Geometry check sheet. Reference: the model listing, model coordinates, mm. A direction names the side the tool comes from. Coordinates: 2 decimals unless noted, no trailing zeros. Write each loop counter-clockwise with the first axis right and the second up, starting at its lowest first coordinate (ties: lowest second). Pieces come first, ordered by that corner, then holes. Notation, with made-up numbers: (-20.75, 72.25) -> (38.25, 72.25) arc R24 cw to (38.25, 105.25) -> close; hole circle Ø4 at (10, -15). An arc over 180 degrees is marked (long way). Answer in a Markdown table with one row per item. Add a question column.
Q1. Thickness scan on line 1 (Z direction, x = 13, y = -44); line 2 (Z direction, x = -9, y = -17); line 3 (X direction, y = -8.5, z = 63). Record the ranges inside material, lowest first.
Q2. Tool access check on faces 1 (the face through (9.934, -49, 29)), 2 (the face through (29.926, -25, 20)), 3 (the face through (-20.112, -49, 12)). Record the directions out of +Z, -Z, +X, -X, +Y, -Y that give a thin tool (end or side, any length) a straight path to the whole face; none if there is none.
Q3. Section check D-D, the plane x = -7. Record the boundary of the cut face in (y, z), and give its area (3 significant figures).
Q4. Section check C-C, the plane z = 60.5. Record the boundary of the cut face in (x, y).
Q5. Release check for a two-part mould opening along Z. For faces 4 (the face through (15.172, -24.65, 54.702)), 5 (the face through (0, -50, 28)), 6 (the face through (13.811, -49, 37)) record: pulls with the +Z half, pulls with the -Z half, needs draft (parallel to the pull), parting line crosses it, or undercut.
Q6. Gauge pin test, flat ends, axial feed: P1, Ø2, axis at x = 17.5, z = 29, coming from the -Y side; P2, Ø1, axis at x = 9, y = -38, coming from the +Z side; P3, Ø1, axis at y = -43.5, z = 62.5, coming from the -X side. Record the tip position at first contact, or that the pin passes through.
Q7. Section check A-A, the plane y = -8. Record the boundary of the cut face in (x, z).
Q8. Section check B-B, the plane x = -18. Record the boundary of the cut face in (y, z), and give its area (3 significant figures).
```python
from build123d import *

# Parameters (mm, degrees)
PAD_DEPTH            = 50
SKETCH001_W          = 14.321759
SKETCH001_H          = 23.338661
POCKET_DEPTH         = 2
SKETCH004_W          = 3.777545
SKETCH004_H          = 5.566906
POCKET001_DEPTH      = 2
SKETCH005_W          = 3.988077
SKETCH005_H          = 5.534469
POCKET002_DEPTH      = 2
SKETCH006_W          = 3.743909
SKETCH006_H          = 5.941416
POCKET003_DEPTH      = 2
SKETCH007_W          = 4.200878
SKETCH007_H          = 5.837583
POCKET004_DEPTH      = 2
BODY_PLACEMENT_ANGLE = 90


with BuildPart() as part:
    # Sketch → Pad (new body)
    with BuildSketch(Plane.XY):
        Polygon((-30.008501, 0), (29.925684, 0), (29.925684, 39.928391), (0, 69.895485), (-30.008501, 40.105713), align=None)
    extrude(amount=PAD_DEPTH)

    # Sketch001 (on Face7 of Pad) → Pocket (cut)
    with BuildSketch(Plane.XY.offset(50)):
        with Locations((-12.951147, 11.66933)):
            Rectangle(SKETCH001_W, SKETCH001_H)
    extrude(amount=-POCKET_DEPTH, mode=Mode.SUBTRACT)

    # Sketch004 (on Face4 of Pocket) → Pocket001 (cut)
    with BuildSketch(Plane.XY.offset(50)):
        with Locations((11.92271, 37.153109)):
            Rectangle(SKETCH004_W, SKETCH004_H)
    extrude(amount=-POCKET001_DEPTH, mode=Mode.SUBTRACT)

    # Sketch005 (on Face4 of Pocket001) → Pocket002 (cut)
    with BuildSketch(Plane.XY.offset(50)):
        with Locations((18.594975, 37.152287)):
            Rectangle(SKETCH005_W, SKETCH005_H)
    extrude(amount=-POCKET002_DEPTH, mode=Mode.SUBTRACT)

    # Sketch006 (on Face4 of Pocket002) → Pocket003 (cut)
    with BuildSketch(Plane.XY.offset(50)):
        with Locations((11.805747, 28.857034)):
            Rectangle(SKETCH006_W, SKETCH006_H)
    extrude(amount=-POCKET003_DEPTH, mode=Mode.SUBTRACT)

    # Sketch007 (on Face4 of Pocket003) → Pocket004 (cut)
    with BuildSketch(Plane.XY.offset(50)):
        with Locations((18.480049, 28.816772)):
            Rectangle(SKETCH007_W, SKETCH007_H)
    extrude(amount=-POCKET004_DEPTH, mode=Mode.SUBTRACT)


with BuildPart() as part_1:
    # Body placement: moved
    add(part.part.rotate(Axis((0, 0, 0), (1, 0, 0)), BODY_PLACEMENT_ANGLE))


solid = part_1.part
```
Calculated:
| question | item | result |
|---|---|---|
| 1 | line 1 | z = 0 to 56.88 |
| 1 | line 2 | z = 0 to 60.96 |
| 1 | line 3 | x = -6.95 to 6.89 |
| 2 | face 1 | -Y |
| 2 | face 2 | +Z, -Z, +X, +Y, -Y |
| 2 | face 3 | -Z, -Y |
| 3 | outline | (-50, 23.34) -> (-48, 23.34) -> (-48, 0) -> (0, 0) -> (0, 62.95) -> (-50, 62.95) -> close |
| 3 | area | 3,100 mm² |
| 4 | outline | (-9.46, -50) -> (9.38, -50) -> (9.38, 0) -> (-9.46, 0) -> close |
| 5 | face 4 | pulls with the +Z half |
| 5 | face 5 | needs draft |
| 5 | face 6 | undercut |
| 6 | P1 | stops at y = -48 |
| 6 | P2 | stops at z = 61.38 |
| 6 | P3 | stops at x = -7.95 |
| 7 | outline | (-30.01, 0) -> (29.93, 0) -> (29.93, 39.93) -> (0, 69.9) -> (-30.01, 40.11) -> close |
| 8 | outline | (-50, 23.34) -> (-48, 23.34) -> (-48, 0) -> (0, 0) -> (0, 52.03) -> (-50, 52.03) -> close |
| 8 | area | 2,550 mm² |
